Work out the finished part from the listing and answer in its coordinate system (mm). A direction names the side the tool comes from. Coordinates: 2 decimals unless noted, no trailing zeros. Write each question's results on one line, items separated by ' | '. Start each with the question number.
1. Find the intervals of material crossed by line 1 along Y through (x, z) = (0, -3); line 2 along Y through (x, z) = (0, 3.9); line 3 along X through (y, z) = (4.5, 0), in increasing order. Write a range as [from, to].
2. Each of these flat-tipped pins is pushed along its axis until it touches: P1, Ø13, axis at x = 12.02, y = -12.02, coming from the -Z side; P2, Ø3.5, axis at x = 0, y = 0, coming from the -Z side; P3, Ø5, axis at x = 1, z = 0.5, coming from the +Y side; P4, Ø1.5, axis at x = -20.5, y = -13.5, coming from the +Z side. Where does it stop, or does it pass through?
3. Which of the six approach directions +Z, -Z, +X, -X, +Y, -Y give full straight-line access (tool end or side, diameter ignored) to faces 1 (the cylindrical face through (-0.07, -1.5, -2.27)), 2 (the cylindrical face through (23.846, 7.509, 3.52))?
4. Determine the mould class of faces 3 (the cylindrical face through (23.846, 7.509, -3.52)), 4 (the cylindrical face through (-29.97, 1.32, 0.07)), 5 (the flat face through (-7, 25, 5)) for opening direction Y: released by +Y, released by -Y, zero draft, split by the parting line, or undercut.
5. A cutting plane is placed at A-A on z = 0.5. State how many separate pieces and enclosed holes the cut face has, then the cut area to 3 significant figures.
from build123d import *

# Parameters (mm, degrees)
SKETCH2_R           = 30
BOSS_EXTRUDE2_DEPTH = 5
SKETCH3_R           = 25
SKETCH3_R_2         = 5
CUT_EXTRUDE1_DEPTH  = 3
SKETCH4_R           = 5
CUT_EXTRUDE2_DEPTH  = 44
CHAMFER1_SIZE       = 0.1


with BuildPart() as part:
    # Sketch2 → Boss-Extrude2 (new, symmetric)
    with BuildSketch(Plane.XY):
        Circle(SKETCH2_R)
    extrude(amount=BOSS_EXTRUDE2_DEPTH, both=True)

    # Sketch3 → Cut-Extrude1 (cut)
    with BuildSketch(Plane.XY.offset(5)):
        Circle(SKETCH3_R)
        Circle(SKETCH3_R_2, mode=Mode.SUBTRACT)
    cut_extrude1 = extrude(amount=-CUT_EXTRUDE1_DEPTH, mode=Mode.SUBTRACT)

    # Mirror1: Cut-Extrude1 across plane
    add(cut_extrude1.mirror(Plane.XY), mode=Mode.SUBTRACT)

    # Sketch4 → Cut-Extrude2 (cut, through all)
    with BuildSketch(Plane.XY.offset(2)):
        with Locations((0, 17)):
            Circle(SKETCH4_R)
        with Locations((12.02081528, 12.02081528)):
            Circle(SKETCH4_R)
        with Locations((17, 0)):
            Circle(SKETCH4_R)
        with Locations((12.02081528, -12.02081528)):
            Circle(SKETCH4_R)
        with Locations((0, -17)):
            Circle(SKETCH4_R)
        with Locations((-12.02081528, -12.02081528)):
            Circle(SKETCH4_R)
        with Locations((-17, 0)):
            Circle(SKETCH4_R)
        with Locations((-12.02081528, 12.02081528)):
            Circle(SKETCH4_R)
    extrude(amount=-CUT_EXTRUDE2_DEPTH, mode=Mode.SUBTRACT)

    # Chamfer1
    chamfer1_edges = [part.edges().sort_by_distance(p)[0] for p in [
        (-25, 0, -2),
        (-5, 0, -5),
        (-25, 0, -5),
        (-30, 0, -5),
        (-17.02081528, 12.02081528, -2),
        (-17.02081528, 12.02081528, 2),
        (-22, 0, -2),
        (-22, 0, 2),
        (-17.02081528, -12.02081528, -2),
        (-17.02081528, -12.02081528, 2),
        (-5, -17, -2),
        (-5, -17, 2),
        (7.02081528, -12.02081528, -2),
        (7.02081528, -12.02081528, 2),
        (12, 0, -2),
        (12, 0, 2),
        (7.02081528, 12.02081528, -2),
        (7.02081528, 12.02081528, 2),
        (-5, 17, -2),
        (-5, 17, 2),
        (-30, 0, 5),
        (-25, 0, 2),
        (-25, 0, 5),
        (-5, 0, 5),
    ]]
    chamfer(chamfer1_edges, length=CHAMFER1_SIZE)

    # Sketch8 → Cut-Revolve1 (revolve, cut)
    with BuildSketch(Plane(origin=(0, 0, 0), x_dir=(0, 0, -1), z_dir=(1, 0, 0))):
        Polygon((-5, 0), (-5, 2), (1, 2), (1, 1.5), (3.5, 1.5), (5, 3), (5, 0), align=None)
    revolve(axis=Axis((0, 0, -5), (0, 0, 1)), mode=Mode.SUBTRACT)


solid = part.part
Values:
1) line 1: [-30, -25], [-5, -1.5], [1.5, 5], [25, 30] | line 2: [-30, -25], [-5, -2], [2, 5], [25, 30] | line 3: [-29.66, -19.18], [-14.82, 14.82], [19.18, 29.66]
2) P1: z = -2 | P2: z = -3.75 | P3: y = 30 | P4: z = 5
3) face 1: +Z, -Z | face 2: +Z
4) face 3: undercut | face 4: split by the parting line | face 5: zero draft
5) separate pieces: 1 | enclosed holes: 9 | area: 2,190 mm^2
